from build123d import *

# Parameters (mm, degrees)
FILLET1_R = 0.4


with BuildPart() as part:
    # Sketch1 → Revolve1 (revolve)
    with BuildSketch(Plane.XY, mode=Mode.PRIVATE) as revolve1_sk:
        with BuildLine():
            Line((5, -2), (5, -5))
            Line((5, -5), (13, -5))
            Line((13, -5), (13, -2))
            Line((13, -2), (11.236067977, -2))
            ThreePointArc((11.236067977, -2), (9, -3), (6.763932023, -2))
            Line((6.763932023, -2), (5, -2))
        make_face()
    revolve(revolve1_sk.sketch.rotate(Axis((0, 5, 0), (0, -1, 0)), 180), axis=Axis((0, 5, 0), (0, -1, 0)))

    # Fillet1
    fillet1_edges = [part.edges().sort_by_distance(p)[0] for p in [
        (13, -2, 0),
        (13, -5, 0),
        (5, -5, 0),
    ]]
    fillet(fillet1_edges, radius=FILLET1_R)


solid = part.part
The model under review builds one solid part; all positions refer to its coordinate system, in mm. Coordinates: 2 decimals unless noted, no trailing zeros. Write each loop counter-clockwise with the first axis right and the second up, starting at its lowest first coordinate (ties: lowest second). Pieces come first, ordered by that corner, then holes. Notation, with made-up numbers: (-34.75, 58.5) -> (-21.75, 58.5) arc R25 ccw to (-21.75, 94.5) -> close; hole circle Ø5 at (62.5, -33.5). An arc over 180 degrees is marked (long way). Answer in a Markdown table with one row per item.
1. Wall thickness on probe 1 along Z at (x, y) = (0, -3.8); probe 2 along Z at (x, y) = (2.75, -2.65); probe 3 along X at (y, z) = (-3.65, -12): over which ranges is each line inside the solid? List them lowest first. Write a range as [from, to].
Answers below:
| item | result |
|---|---|
| probe 1 | z = [-13, -5], [5, 13] |
| probe 2 | z = [-12.71, -10.04], [-7.08, -4.18], [4.18, 7.08], [10.04, 12.71] |
| probe 3 | x = [-5, 5] |
2. We need section A-A, the plane x = 0. State the section outline as (y, z) points.
Answers below:
| item | result |
|---|---|
| outline | (-5, -12.6) arc R0.4 ccw to (-4.6, -13) -> (-2.4, -13) arc R0.4 ccw to (-2, -12.6) -> (-2, -11.24) arc R3 cw to (-2, -6.76) -> (-2, -5) -> (-4.6, -5) arc R0.4 ccw to (-5, -5.4) -> close; (-5, 5.4) arc R0.4 ccw to (-4.6, 5) -> (-2, 5) -> (-2, 6.76) arc R3 cw to (-2, 11.24) -> (-2, 12.6) arc R0.4 ccw to (-2.4, 13) -> (-4.6, 13) arc R0.4 ccw to (-5, 12.6) -> close |
3. We need section B-B, the plane z = 0. State the section outline as (x, y) points, and give its area (3 significant figures).
Answers below:
| item | result |
|---|---|
| outline | (-13, -4.6) arc R0.4 ccw to (-12.6, -5) -> (-5.4, -5) arc R0.4 ccw to (-5, -4.6) -> (-5, -2) -> (-6.76, -2) arc R3 cw to (-11.24, -2) -> (-12.6, -2) arc R0.4 ccw to (-13, -2.4) -> close; (5, -4.6) arc R0.4 ccw to (5.4, -5) -> (12.6, -5) arc R0.4 ccw to (13, -4.6) -> (13, -2.4) arc R0.4 ccw to (12.6, -2) -> (11.24, -2) arc R3 cw to (6.76, -2) -> (5, -2) -> close |
| area | 41.6 mm^2 |
4. We need section C-C, the plane y = -3.95. State the section outline as (x, z) points, and give its area (3 significant figures).
Answers below:
| item | result |
|---|---|
| outline | circle Ø26 at (0, 0); hole circle Ø10 at (0, 0) |
| area | 452 mm^2 |
5. Draft analysis for pull direction Z (two halves, no side actions). For faces 1 (the cylindrical face through (5, -3, 0)), 2 (the flat face through (11.3, -2, 1.8)), 3 (the cylindrical face through (10.316, -3.485, 7.91)), state which applies: +Z half, -Z half, draft (parallel to the pull), parting line (faces both ways), or undercut.
Answers below:
| item | result |
|---|---|
| face 1 | undercut |
| face 2 | draft |
| face 3 | parting line |
6. Clearance check with flat-ended pins moving along their axes: pin 1 Ø1 at (x, y) = (7.5, -3) entering from -Z; pin 2 Ø1 at (x, z) = (-8.5, 2.5) entering from +Y; pin 3 Ø1.5 at (y, z) = (-2.5, -3.5) entering from -X. State where each tip first meets the part, or that it passes through.
Answers below:
| item | result |
|---|---|
| pin 1 | stops at z = -10.95 |
| pin 2 | stops at y = -2.93 |
| pin 3 | stops at x = -12.71 |
